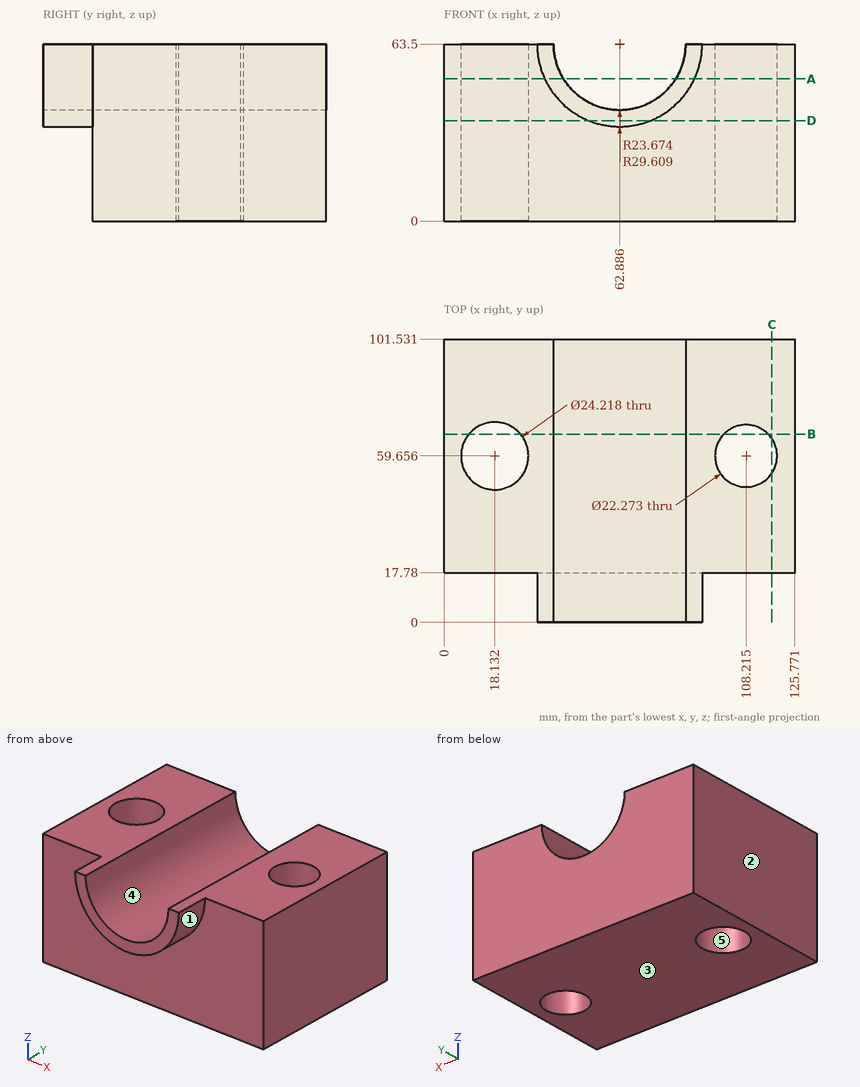
Verification items for this drawing (mm, ordinates from the low corner). A direction names the side the tool comes from. Round coordinates to 2 decimals unless told otherwise and drop trailing zeros. Loops run counter-clockwise (first coordinate to the right, second up) from the corner with the lowest first, then second, coordinate; pieces in that order, holes last. Notation, with made-up numbers: (42.5, 73) -> (46.5, 73) arc R10 cw to (46.5, 89) -> close; hole circle Ø5 at (-9.75, 44). An arc over 180 degrees is marked (long way). Answer in a Markdown table with one row per item.
Q1. Sectioned sample at B-B on y = 67.5. Enter the section's corners in (x, z) (1 decimal), then the cut area to 3 significant figures.
Data:
| item | result |
|---|---|
| outline | (0, 0) -> (8.9, 0) -> (8.9, 63.5) -> (0, 63.5) -> close; (27.4, 0) -> (100.3, 0) -> (100.3, 63.5) -> (86.6, 63.5) arc R23.7 cw to (39.2, 63.5) -> (27.4, 63.5) -> close; (116.1, 0) -> (125.8, 0) -> (125.8, 63.5) -> (116.1, 63.5) -> close |
| area | 4,930 mm^2 |
Q2. Release check for a two-part mould opening along Z. For the marked faces 3, 4 and 5 record: released by +Z, released by -Z, zero draft, split by the parting line, or undercut.
Data:
| item | result |
|---|---|
| face 3 | released by -Z |
| face 4 | released by +Z |
| face 5 | zero draft |
Q3. Sectioned sample at C-C on x = 117.5. Enter the section's corners in (y, z) (1 decimal).
Data:
| item | result |
|---|---|
| outline | (17.8, 0) -> (53.5, 0) -> (53.5, 63.5) -> (17.8, 63.5) -> close; (65.8, 0) -> (101.5, 0) -> (101.5, 63.5) -> (65.8, 63.5) -> close |
Q4. Sectioned sample at A-A on z = 51. Enter the section's corners in (x, y) (1 decimal).
Data:
| item | result |
|---|---|
| outline | (0, 17.8) -> (36, 17.8) -> (36, 0) -> (42.8, 0) -> (42.8, 101.5) -> (0, 101.5) -> close; (83, 0) -> (89.7, 0) -> (89.7, 17.8) -> (125.8, 17.8) -> (125.8, 101.5) -> (83, 101.5) -> close; hole circle Ø24.2 at (18.1, 59.7); hole circle Ø22.3 at (108.2, 59.7) |
Q5. Sectioned sample at D-D on z = 36. Enter the section's corners in (x, y) (1 decimal), then the cut area to 3 significant figures.
Data:
| item | result |
|---|---|
| outline | (0, 17.8) -> (51.9, 17.8) -> (51.9, 0) -> (73.9, 0) -> (73.9, 17.8) -> (125.8, 17.8) -> (125.8, 101.5) -> (0, 101.5) -> close; hole circle Ø24.2 at (18.1, 59.7); hole circle Ø22.3 at (108.2, 59.7) |
| area | 10,100 mm^2 |
Q6. Thickness scan on L1, parallel to X at y = 60.5, z = 37; L2, parallel to Y at x = 108.5, z = 8.5; L3, parallel to X at y = 58.5, z = 45 (1 decimal). Record the ranges inside material, lowest first.
Data:
| item | result |
|---|---|
| L1 | x = 0 to 6.05, 30.21 to 97.11, 119.32 to 125.77 |
| L2 | y = 17.78 to 48.52, 70.79 to 101.53 |
| L3 | x = 0 to 6.1, 30.2 to 48.1, 77.7 to 97.1, 119.3 to 125.8 |
Q7. Go/stop test with flat-tipped pins: P1, Ø4, axis at x = 79.5, y = 63.5, coming from the +Z side; P2, Ø3, axis at x = 26, z = 33, coming from the -Y side. Record where each tip stops, or that it passes through.
Data:
| item | result |
|---|---|
| P1 | stops at z = 48.87 |
| P2 | stops at y = 17.78 |
Q8. Set-up check for the marked faces 1 and 2: record each of +Z, -Z, +X, -X, +Y, -Y from which the full face is reachable in a straight line by a thin tool's end or side.
Data:
| item | result |
|---|---|
| face 1 | -Z, -Y |
| face 2 | +Z, -Z, -X, +Y, -Y |
